For this review, take the finished solid that the model builds, in its own axes (mm). Face numbers are marked on the shaded views. A direction names the side the tool comes from. Give positions to 0.01 mm unless a question says otherwise; leave off trailing zeros. Write each loop counter-clockwise with the first axis right and the second up, starting at its lowest first coordinate (ties: lowest second). Pieces come first, ordered by that corner, then holes. Notation, with made-up numbers: M -12,-20 L 5,-20 A31 ccw 5,18 Z; hole C -32.75,-22.75 d6. An arc over 180 degrees is marked long. Answer as a JSON object with one key per item and string values. Group by question number.
```python
from build123d import *

# Parameters (mm, degrees)
SKIZZE1_W                       = 55
SKIZZE1_H                       = 40
SKIZZE1_R                       = 1.35
AUFSATZ_LINEAR_AUSTRAGEN1_DEPTH = 5.6
SKIZZE2_W                       = 33.875763277
SKIZZE2_H                       = 6.167598205
SKIZZE2_W_2                     = 6.167598205
SKIZZE2_H_2                     = 21.172352048
AUFSATZ_LINEAR_AUSTRAGEN2_DEPTH = 8.5
SKIZZE2_3_W                     = 9.48153157
SKIZZE2_3_H                     = 8.400032762
AUFSATZ_LINEAR_AUSTRAGEN3_DEPTH = 4
SKIZZE2_4_W                     = 10.217961205
SKIZZE2_4_H                     = 10.125907501
SKIZZE2_4_W_2                   = 10.171934354
SKIZZE2_4_W_3                   = 10.770283433
AUFSATZ_LINEAR_AUSTRAGEN4_DEPTH = 5
SKIZZE2_5_W                     = 22.184942798
SKIZZE2_5_H                     = 9.573585274
AUFSATZ_LINEAR_AUSTRAGEN5_DEPTH = 12.5
SKIZZE2_6_W                     = 24.578339117
SKIZZE2_6_H                     = 7.364296365
AUFSATZ_LINEAR_AUSTRAGEN6_DEPTH = 14
SKIZZE2_7_W                     = 9.113316751
SKIZZE2_7_H                     = 4.418577819
AUFSATZ_LINEAR_AUSTRAGEN7_DEPTH = 2
FASE1_SIZE                      = 4
FASE1_SIZE2                     = 1.865230633
FASE1_PART_2_SIZE               = 4
FASE1_PART_2_SIZE2              = 1.865230633


with BuildPart() as part:
    # Skizze1 → Aufsatz-Linear austragen1 (new body)
    with BuildSketch(Plane(origin=(0, 0, 0), x_dir=(1, 0, 0), z_dir=(0, 1, 0))):
        Rectangle(SKIZZE1_W, SKIZZE1_H)
        with Locations((-23.5, 16)):
            Circle(SKIZZE1_R, mode=Mode.SUBTRACT)
        with Locations((23.5, -16)):
            Circle(SKIZZE1_R, mode=Mode.SUBTRACT)
    extrude(amount=AUFSATZ_LINEAR_AUSTRAGEN1_DEPTH)

    # Skizze2 → Aufsatz-Linear austragen2 (add)
    with BuildSketch(Plane(origin=(0, 5.6, 0), x_dir=(1, 0, 0), z_dir=(0, 1, 0))):
        with Locations((8.681351592, 16.246278391)):
            Rectangle(SKIZZE2_W, SKIZZE2_H)
        with Locations((24.008293401, -2.394596782)):
            Rectangle(SKIZZE2_W_2, SKIZZE2_H_2)
    extrude(amount=AUFSATZ_LINEAR_AUSTRAGEN2_DEPTH)

    # Skizze2<3> → Aufsatz-Linear austragen3 (add)
    with BuildSketch(Plane(origin=(0, 5.6, 0), x_dir=(1, 0, 0), z_dir=(0, 1, 0))):
        with Locations((-20.913914423, -15.799983619)):
            Rectangle(SKIZZE2_3_W, SKIZZE2_3_H)
    extrude(amount=AUFSATZ_LINEAR_AUSTRAGEN3_DEPTH)

    # Skizze2<4> → Aufsatz-Linear austragen4 (add)
    with BuildSketch(Plane(origin=(0, 5.6, 0), x_dir=(1, 0, 0), z_dir=(0, 1, 0))):
        with Locations((-9.591308763, 7.178988492)):
            Rectangle(SKIZZE2_4_W, SKIZZE2_4_H)
        with Locations((2.260605699, 7.178988492)):
            Rectangle(SKIZZE2_4_W_2, SKIZZE2_4_H)
        with Locations((14.066493309, 7.178988492)):
            Rectangle(SKIZZE2_4_W_3, SKIZZE2_4_H)
    extrude(amount=AUFSATZ_LINEAR_AUSTRAGEN4_DEPTH)

    # Skizze2<5> → Aufsatz-Linear austragen5 (add)
    with BuildSketch(Plane(origin=(0, 5.6, 0), x_dir=(1, 0, 0), z_dir=(0, 1, 0))):
        with Locations((7.346572876, -5.524422737)):
            Rectangle(SKIZZE2_5_W, SKIZZE2_5_H)
    extrude(amount=AUFSATZ_LINEAR_AUSTRAGEN5_DEPTH)

    # Skizze2<6> → Aufsatz-Linear austragen6 (add)
    with BuildSketch(Plane(origin=(0, 5.6, 0), x_dir=(1, 0, 0), z_dir=(0, 1, 0))):
        with Locations((7.806841398, -15.282115421)):
            Rectangle(SKIZZE2_6_W, SKIZZE2_6_H)
    extrude(amount=AUFSATZ_LINEAR_AUSTRAGEN6_DEPTH)

    # Skizze2<7> → Aufsatz-Linear austragen7 (add)
    with BuildSketch(Plane(origin=(0, 5.6, 0), x_dir=(1, 0, 0), z_dir=(0, 1, 0))):
        with Locations((-10.14363099, -15.190061716)):
            Rectangle(SKIZZE2_7_W, SKIZZE2_7_H)
    extrude(amount=AUFSATZ_LINEAR_AUSTRAGEN7_DEPTH)

    # Fase1
    fase1_edges = [part.edges().sort_by_distance(p)[0] for p in [
        (8.681351592, 14.1, -19.330077493),
    ]]
    fase1_side = [part.faces().sort_by_distance(p)[0] for p in [
        (8.681351592, 9.85, -19.330077493),
    ]]
    chamfer(fase1_edges, length=FASE1_SIZE, length2=FASE1_SIZE2, reference=fase1_side[0])

    # Fase1 part 2
    fase1_part_2_edges = [part.edges().sort_by_distance(p)[0] for p in [
        (27.092092503, 14.1, 2.394596782),
    ]]
    fase1_part_2_side = [part.faces().sort_by_distance(p)[0] for p in [
        (27.092092503, 9.85, 2.394596782),
    ]]
    chamfer(fase1_part_2_edges, length=FASE1_PART_2_SIZE, length2=FASE1_PART_2_SIZE2, reference=fase1_part_2_side[0])


solid = part.part
```
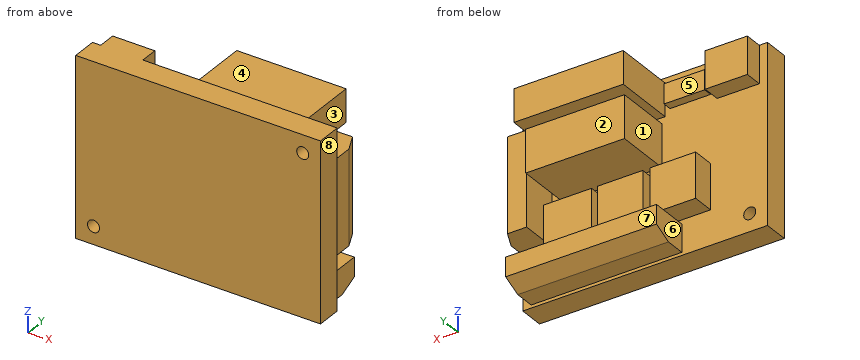
Item 1: Consider section A-A (y = 17.25). Give the boundary of the cut face in (x, z), plus the area to 3 significant figures.
Item 2: Insertion check: P1, Ø8, axis at x = 14.5, z = -9, coming from the +Y side; P2, Ø7, axis at x = 8.5, y = 10, coming from the -Z side; P3, Ø2.5, axis at x = 5.5, y = 12, coming from the +Z side. Each pin has a flat end and moves straight along its axis. Give the tip position at first contact, or say it passes through.
Item 3: Consider section D-D (z = 9). Give the boundary of the cut face in (x, y).
Item 4: To check wall thickness, follow probe 1 along X at (y, z) = (7.75, -10.5); probe 2 along Z at (x, y) = (-23.5, 2.65); probe 3 along X at (y, z) = (9, 13.5). State the ranges of each line that lie inside material, in increasing order.
Item 5: Consider section B-B (x = -23.5). Give the boundary of the cut face in (y, z).
Item 6: Machinability: for the marked faces 1, 2, 3 and 4, which of the approach directions +Z, -Z, +X, -X, +Y, -Y give a long, thin tool a straight path to every point of the face, cutting with its end or side? Answer none if there is none.
Item 7: Draft analysis for pull direction X (two halves, no side actions). For the marked faces 5, 6, 7 and 8, state which applies: released by +X, released by -X, zero draft, split by the parting line, or undercut.
Item 8: Consider section C-C (z = -16). Give the boundary of the cut face in (x, y).
Result set:
{
 "1": {"outline": "M -4.48,11.6 L 20.1,11.6 L 20.1,18.96 L -4.48,18.96 Z; M -3.75,0.74 L 18.44,0.74 L 18.44,10.31 L -3.75,10.31 Z", "area": "393 mm^2"},
 "2": {"P1": "stops at y = 10.6", "P2": "stops at z = -19.33", "P3": "stops at z = 18.96"},
 "3": {"outline": "M -27.5,0 L 27.5,0 L 27.5,5.6 L 27.09,5.6 L 27.09,10.1 L 25.23,14.1 L 20.92,14.1 L 20.92,5.6 L 18.44,5.6 L 18.44,18.1 L -3.75,18.1 L -3.75,5.6 L -27.5,5.6 Z"},
 "4": {"probe 1": "x = -14.7 to -4.48, -2.83 to 7.35, 8.68 to 19.45", "probe 2": "z = -20 to -17.35, -14.65 to 20", "probe 3": "x = -25.65 to -16.17, -4.48 to 20.1"},
 "5": {"outline": "M 0,-20 L 5.6,-20 L 5.6,-17.35 L 0,-17.35 Z; M 0,-14.65 L 5.6,-14.65 L 5.6,11.6 L 9.6,11.6 L 9.6,20 L 0,20 Z"},
 "6": {"face 1": "-X, +Y", "face 2": "-Z, +X, -X, +Y", "face 3": "+Z, +Y", "face 4": "+Z, +X, +Y"},
 "7": {"face 5": "undercut", "face 6": "released by -X", "face 7": "zero draft", "face 8": "released by +X"},
 "8": {"outline": "M -27.5,0 L -24.85,0 L -24.85,5.6 L -27.5,5.6 Z; M -22.15,0 L 27.5,0 L 27.5,5.6 L 25.62,5.6 L 25.62,14.1 L -8.26,14.1 L -8.26,5.6 L -22.15,5.6 Z"}
}
